from build123d import *

# Parameters (mm, degrees)
F0_R     = 2.5
F1_DEPTH = 3


with BuildPart() as f1:
    # F0 (on Front) → F1 (new body)
    with BuildSketch(Plane.XZ):
        with BuildLine():
            Line((8.5, 0), (0, 0))
            Line((0, 0), (0, -65))
            Line((0, -65), (35, -65))
            Line((35, -65), (41, -65.5))
            Line((41, -65.5), (57, -69.5))
            Line((57, -69.5), (212, -129.5))
            Line((212, -129.5), (234, -129.5))
            Line((234, -129.5), (234, -128))
            Line((234, -128), (234.5, -128))
            Line((234.5, -128), (240, -129.5))
            Line((240, -129.5), (250, -129.5))
            Line((250, -129.5), (253, -118.5))
            ThreePointArc((253, -118.5), (251.054419, -79), (253, -39.5))
            Line((253, -39.5), (253, -26.5))
            Line((253, -26.5), (251.5, -25))
            Line((251.5, -25), (241.5, -25))
            Line((241.5, -25), (235.5, -27.5))
            Line((235.5, -27.5), (234.5, -27.5))
            Line((234.5, -27.5), (234.5, -27))
            Line((234.5, -27), (234, -25))
            Line((234, -25), (194.5, -25))
            Line((194.5, -25), (183, -26.5))
            Line((183, -26.5), (77, -26.5))
            Line((77, -26.5), (63.5, -25))
            Line((63.5, -25), (42.5, -19))
            Line((42.5, -19), (34.5, -15))
            Line((34.5, -15), (14.5, -2.5))
            ThreePointArc((14.5, -2.5), (11.60261, -1.003737), (8.5, 0))
        make_face()
        with Locations((215, -113)):
            Circle(F0_R, mode=Mode.SUBTRACT)
        with BuildLine():
            Line((77, -41.5), (87, -41.5))
            Line((87, -41.5), (113, -41.5))
            Line((113, -41.5), (138, -41.5))
            Line((138, -41.5), (180, -41.5))
            Line((180, -41.5), (197, -32))
            Line((197, -32), (217, -32))
            ThreePointArc((217, -32), (218.810814, -33.349419), (219.5, -35.5))
            Line((219.5, -35.5), (219.5, -95.5))
            Line((219.5, -95.5), (216, -103.5))
            ThreePointArc((216, -103.5), (209.345929, -105.300553), (205.636229, -111.110611))
            Line((205.636229, -111.110611), (200, -113.524611))
            Line((200, -113.524611), (145.5, -92.427837))
            Line((145.5, -92.427837), (102.5, -77.5))
            Line((102.5, -77.5), (87, -71.5))
            Line((87, -71.5), (50.5, -59))
            Line((50.5, -59), (43.5, -57.5))
            ThreePointArc((43.5, -57.5), (41.280596, -56.601046), (39.5, -55))
            Line((39.5, -55), (39.5, -40))
            ThreePointArc((39.5, -40), (40.671573, -37.171573), (43.5, -36))
            Line((43.5, -36), (60, -40))
            Line((60, -40), (72, -41.5))
            Line((72, -41.5), (77, -41.5))
        make_face(mode=Mode.SUBTRACT)
    extrude(amount=F1_DEPTH)


solid = f1.part
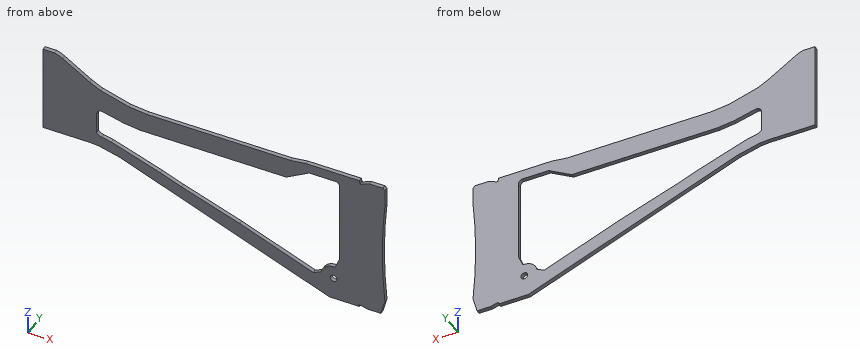
For this review, take the finished solid that the model builds, in its own axes (mm). Give positions to 0.01 mm unless a question says otherwise; leave off trailing zeros. Loops run counter-clockwise (first coordinate to the right, second up) from the corner with the lowest first, then second, coordinate; pieces in that order, holes last.
Item 1: Insertion check: pin 1 (1 mm diameter, centred on x = 189, y = -2.5, fed in from +Z); pin 2 (3 mm diameter, centred on x = 215, z = -113, fed in from -Y); pin 3 (1 mm diameter, centred on y = -0.5, z = -71, fed in from +X); pin 4 (1.5 mm diameter, centred on x = 245, y = -1.5, fed in from +Z). Each pin has a flat end and moves straight along its axis. Give the tip position at first contact, or say it passes through.
Item 2: Take a section at D-D, the plane z = -10.5. State the section outline as (x, y) points.
Item 3: Take a section at C-C, the plane y = -2.35. Give the number of separate pieces and of enclosed holes in the cut face, and give its area (3 significant figures).
Item 4: Take a section at A-A, the plane z = -48. State the section outline as (x, y) points, and give its area (3 significant figures).
Item 5: Take a section at B-B, the plane x = 168. State the section outline as (y, z) points.
Item 6: For line 1 along Z through (x, y) = (215, -1.55); line 2 along Z through (x, y) = (113, -1); line 3 along Z through (x, y) = (107, -1.75), list the stretches that pass through material, from the lowest coordinate up.
Calculated:
1. pin 1: stops at z = -25.65
1. pin 2: passes through
1. pin 3: stops at x = 251.14
1. pin 4: stops at z = -25
2. outline: (0, -3) - (27.3, -3) - (27.3, 0) - (0, 0) - close
3. separate pieces: 1
3. enclosed holes: 2
3. area: 10,200 mm2
4. outline: (0, -3) - (39.5, -3) - (39.5, 0) - (0, 0) - close; (219.5, -3) - (252.25, -3) - (252.25, 0) - (219.5, 0) - close
4. area: 217 mm2
5. outline: (-3, -112.47) - (0, -112.47) - (0, -101.14) - (-3, -101.14) - close; (-3, -41.5) - (0, -41.5) - (0, -26.5) - (-3, -26.5) - close
6. line 1: z = -129.5 to -115.5, -110.5 to -103.45, -32 to -25
6. line 2: z = -91.18 to -81.15, -41.5 to -26.5
6. line 3: z = -88.85 to -79.06, -41.5 to -26.5
